Design review of the part built by this model. Coordinates are the model's own, in mm. A direction names the side the tool comes from. Round coordinates to 2 decimals unless told otherwise and drop trailing zeros. Order: outer loops, then holes, each group sorted by start corner. A loop starts at its lowest first (then second) coordinate and runs counter-clockwise, first axis right, second up. Notation, with made-up numbers: M 34.25,87.25 L 71.25,87.25 A10 cw 71.25,94.25 Z; hole C 62,5.5 d9. An arc over 180 degrees is marked long. Write each question's results on one line, items separated by ' | '. Start each with the question number.
Item 1: Take a section at D-D, the plane z = 22.75. Write out the cut boundary in (x, y), plus the area to 3 significant figures.
Item 2: Wall thickness on line 1 (X direction, y = -44, z = 7); line 2 (X direction, y = 24.5, z = 11); line 3 (Y direction, x = 12.7, z = 11): over which ranges is each line inside the solid? List them lowest first. Write a range as [from, to].
Item 3: The part is to be moulded in two halves that separate along Y. For faces 1 (the flat face through (25.4, -54, 13)), 2 (the cylindrical face through (-12.878, -86.248, 14.607)), 3 (the flat face through (37.92, -89.76, 3.22)), 4 (the cylindrical face through (37.922, -86.248, 14.607)), say which applies: +Y half, -Y half, draft (parallel to the pull), parting line (faces both ways), or undercut.
Item 4: Take a section at A-A, the plane x = 12.7. Write out the cut boundary in (y, z).
Item 5: Take a section at C-C, the plane z = 12.7. Write out the cut boundary in (x, y).
Item 6: Take a section at B-B, the plane y = -51.5. Write out the cut boundary in (x, z), plus the area to 3 significant figures.
Item 7: Clearance check with flat-ended pins moving along their axes: pin 1 (7.5 mm diameter, centred on y = 59.5, z = 19, fed in from -X); pin 2 (14.5 mm diameter, centred on x = 12.7, y = 72.21, fed in from +Z); pin 3 (2 mm diameter, centred on x = 29, z = 8, fed in from +Y); pin 4 (3 mm diameter, centred on y = 61.5, z = 22.5, fed in from +X). State where each tip first meets the part, or that it passes through.
Item 8: Machinability: for faces 5 (the flat face through (0, 54, 13)), 6 (the flat face through (25.4, 53, 13)), 7 (the flat face through (50.8, -49, 13)), which of the approach directions +Z, -Z, +X, -X, +Y, -Y give a long, thin tool a straight path to every point of the face, cutting with its end or side? Answer none if there is none.
```python
from build123d import *

# Parameters (mm, degrees)
F0_R     = 6.35
F1_DEPTH = 25.4
F2_R     = 6.35
F3_DEPTH = 76.2
F4_SIZE  = 6.35


with BuildPart() as f1:
    # F0 (on Top) → F1 (new body)
    with BuildSketch(Plane.XY):
        with BuildLine():
            Line((25.4, 84.908329), (0, 84.908329))
            Line((0, 84.908329), (0, 21.408329))
            ThreePointArc((0, 21.408329), (-3.719744, 12.428073), (-12.7, 8.708329))
            ThreePointArc((-12.7, 8.708329), (-21.680256, 4.988585), (-25.4, -3.991671))
            Line((-25.4, -3.991671), (-25.4, -92.891671))
            Line((-25.4, -92.891671), (0, -92.891671))
            Line((0, -92.891671), (0, -16.691671))
            ThreePointArc((0, -16.691671), (12.7, -3.991671), (25.4, -16.691671))
            Line((25.4, -16.691671), (25.4, -92.891671))
            Line((25.4, -92.891671), (50.8, -92.891671))
            Line((50.8, -92.891671), (50.8, -3.991671))
            ThreePointArc((50.8, -3.991671), (47.080256, 4.988585), (38.1, 8.708329))
            ThreePointArc((38.1, 8.708329), (29.119744, 12.428073), (25.4, 21.408329))
            Line((25.4, 21.408329), (25.4, 84.908329))
        make_face()
        with Locations((12.7, 72.208329)):
            Circle(F0_R, mode=Mode.SUBTRACT)
    extrude(amount=F1_DEPTH)

    # F2 (on face) → F3 (cut)
    with BuildSketch(Plane(origin=(-25.4, 0, 0), x_dir=(0, -1, 0), z_dir=(-1, 0, 0))):
        with Locations((80.191671, 12.7)):
            Circle(F2_R)
    extrude(amount=-F3_DEPTH, mode=Mode.SUBTRACT)

    # F4
    f4_edges = [f1.edges().sort_by_distance(p)[0] for p in [
        (-12.7, -92.891671, 25.4),
        (-12.7, -92.891671, 0),
        (38.1, -92.891671, 25.4),
        (38.1, -92.891671, 0),
    ]]
    chamfer(f4_edges, length=F4_SIZE)


solid = f1.part
```
Results list:
1) outline: M -25.4,-89.19 L 0,-89.19 L 0,-16.69 A12.7 cw 25.4,-16.69 L 25.4,-89.19 L 50.8,-89.19 L 50.8,-3.99 A12.7 ccw 38.1,8.71 A12.7 cw 25.4,21.41 L 25.4,84.91 L 0,84.91 L 0,21.41 A12.7 cw -12.7,8.71 A12.7 ccw -25.4,-3.99 Z; hole C 12.7,72.21 d12.7 | area: 7,170 mm²
2) line 1: [-25.4, 0], [25.4, 50.8] | line 2: [0, 25.4] | line 3: [-3.99, 65.86], [78.56, 84.91]
3) face 1: draft | face 2: undercut | face 3: -Y half | face 4: undercut
4) outline: M -3.99,0 L 65.86,0 L 65.86,25.4 L -3.99,25.4 Z; M 78.56,0 L 84.91,0 L 84.91,25.4 L 78.56,25.4 Z
5) outline: M -25.4,-92.89 L 0,-92.89 L 0,-86.54 L -25.4,-86.54 Z; M -25.4,-73.84 L 0,-73.84 L 0,-16.69 A12.7 cw 25.4,-16.69 L 25.4,-73.84 L 50.8,-73.84 L 50.8,-3.99 A12.7 ccw 38.1,8.71 A12.7 cw 25.4,21.41 L 25.4,84.91 L 0,84.91 L 0,21.41 A12.7 cw -12.7,8.71 A12.7 ccw -25.4,-3.99 Z; M 25.4,-92.89 L 50.8,-92.89 L 50.8,-86.54 L 25.4,-86.54 Z; hole C 12.7,72.21 d12.7
6) outline: M -25.4,0 L 0,0 L 0,25.4 L -25.4,25.4 Z; M 25.4,0 L 50.8,0 L 50.8,25.4 L 25.4,25.4 Z | area: 1,290 mm²
7) pin 1: x = 0 | pin 2: z = 25.4 | pin 3: y = 13.71 | pin 4: x = 25.4
8) face 5: +Z, -Z, -X, +Y | face 6: +Z, -Z, +X, +Y | face 7: +Z, -Z, +X, +Y, -Y
